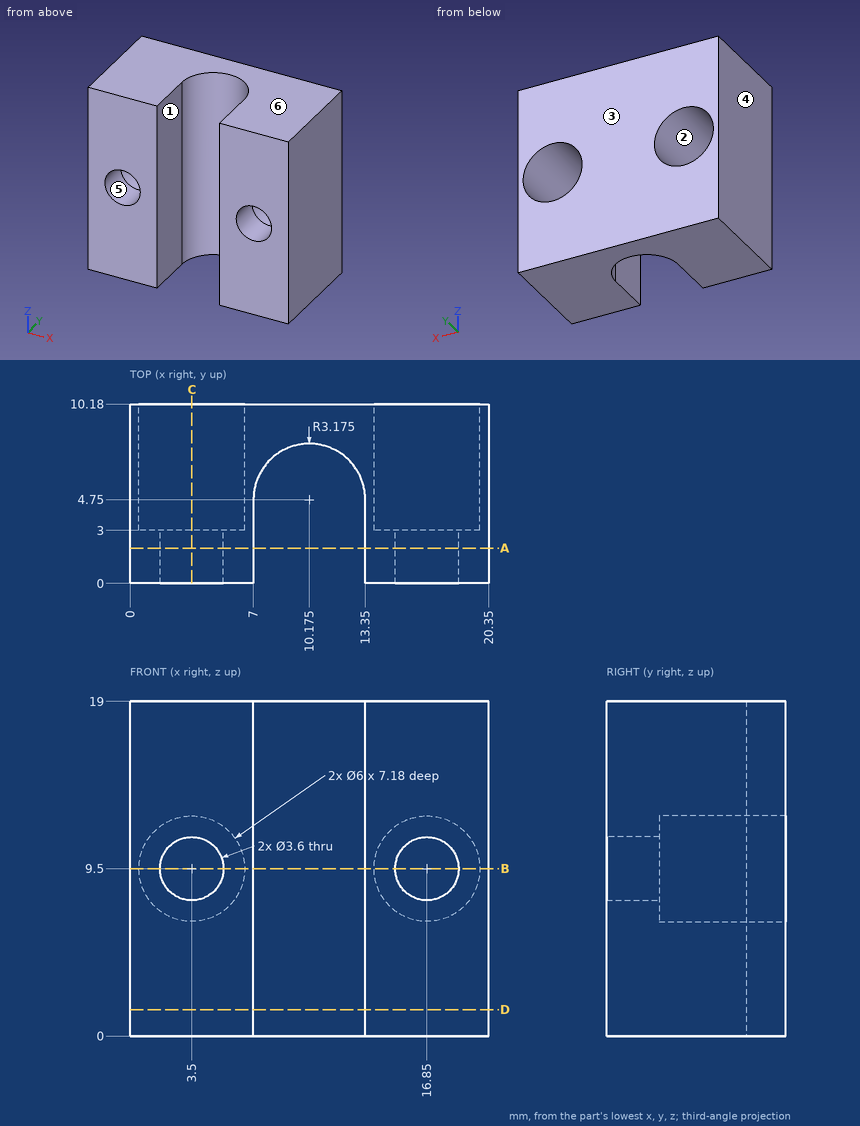
Source: three-view drawing plus pictorial views. Frame: mm from the lowest corner of the part. A direction names the side the tool comes from. Round coordinates to 2 decimals unless told otherwise and drop trailing zeros. Loops run counter-clockwise (first coordinate to the right, second up) from the corner with the lowest first, then second, coordinate; pieces in that order, holes last. Notation, with made-up numbers: M -20,76 L 36,76 A15 ccw 36,100 Z; hole C 64,56 d8. An arc over 180 degrees is marked long. Answer as CSV lines item,"result". Start each with the question number.
(1) Draft query along Z for the marked faces 4, 5 and 6. Return one class per face: released by +Z, released by -Z, zero draft, split by the parting line, or undercut.
(2) Section C-C, the plane x = 3.5. Output: boundary loops of the cut face in (y, z).
(3) Line query: line 1 (X direction, y = 1.15, z = 9.5); line 2 (X direction, y = 1.75, z = 5.75); line 3 (X direction, y = 6.5, z = 8). Output: solid intervals per line, ascending. Write a range as [from, to].
(4) First-contact query: pin 1 (3 mm diameter, centred on x = 4.5, z = 10, fed in from +Y); pin 2 (3.5 mm diameter, centred on x = 3.5, z = 9.5, fed in from -Y). Flat tips, straight axial feed; report the tip coordinate or a pass-through.
(5) Section B-B, the plane z = 9.5. Output: boundary loops of the cut face in (x, y) (3 decimals).
(6) Section A-A, the plane y = 2. Output: boundary loops of the cut face in (x, z).
(7) Section D-D, the plane z = 1.5. Output: boundary loops of the cut face in (x, y) (3 decimals).
(8) Reachability of the marked faces 1, 2 and 3 from +Z, -Z, +X, -X, +Y, -Y: full face, straight path, thin tool, end or side. Return the list, or none.
Values found:
1,face 4,"zero draft"
1,face 5,"undercut"
1,face 6,"released by +Z"
2,outline,"M 0,0 L 10.18,0 L 10.18,6.5 L 3,6.5 L 3,7.7 L 0,7.7 Z; M 0,11.3 L 3,11.3 L 3,12.5 L 10.18,12.5 L 10.18,19 L 0,19 Z"
3,line 1,"x = [0, 1.7], [5.3, 7], [13.35, 15.05], [18.65, 20.35]"
3,line 2,"x = [0, 7], [13.35, 20.35]"
3,line 3,"x = [0, 0.9], [6.1, 7.53], [12.82, 14.25], [19.45, 20.35]"
4,pin 1,"stops at y = 3"
4,pin 2,"passes through"
5,outline,"M 0,0 L 1.7,0 L 1.7,3 L 0.5,3 L 0.5,10.18 L 0,10.18 Z; M 5.3,0 L 7,0 L 7,4.75 A3.175 cw 13.35,4.75 L 13.35,0 L 15.05,0 L 15.05,3 L 13.85,3 L 13.85,10.18 L 6.5,10.18 L 6.5,3 L 5.3,3 Z; M 18.65,0 L 20.35,0 L 20.35,10.18 L 19.85,10.18 L 19.85,3 L 18.65,3 Z"
6,outline,"M 0,0 L 7,0 L 7,19 L 0,19 Z; M 13.35,0 L 20.35,0 L 20.35,19 L 13.35,19 Z; hole C 3.5,9.5 d3.6; hole C 16.85,9.5 d3.6"
7,outline,"M 0,0 L 7,0 L 7,4.75 A3.175 cw 13.35,4.75 L 13.35,0 L 20.35,0 L 20.35,10.18 L 0,10.18 Z"
8,face 1,"+Z, -Z, -Y"
8,face 2,"+Y"
8,face 3,"+Z, -Z, +X, -X, +Y"
